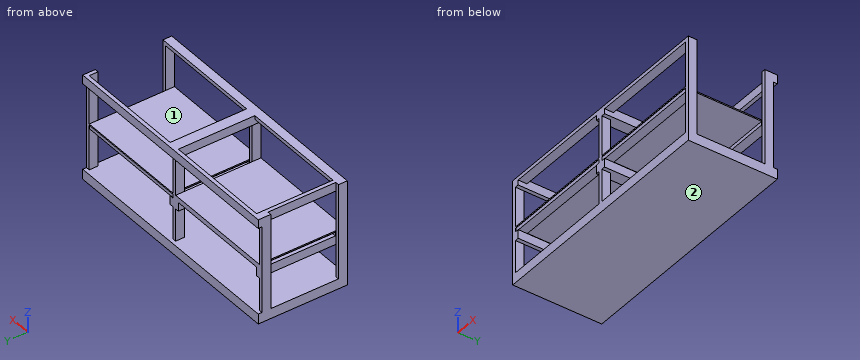
from build123d import *

# Parameters (mm, degrees)
F0_W           = 38.1
F0_H           = 88.9
F1_DEPTH       = 101.6
F2_DEPTH       = 927.1
F3_W           = 2438.4
F3_H           = 88.9
F4_DEPTH       = 38.1
F5_DEPTH       = 965.2
F6_W           = 2438.4
F6_H           = 88.9
F7_DEPTH       = 38.1
F8_W           = 88.9
F8_H           = 50.8
F9_DEPTH       = 38.1
F8_H_2         = 38.1
F8_W_2         = 3.175
F8_W_3         = 85.725
F10_DEPTH      = 1162.05
F11_W          = 863.6
F11_H          = 88.9
F12_DEPTH      = 38.1
F12_DEPTH_BACK = 76.2
F13_W          = 88.9
F13_H          = 38.1
F14_DEPTH      = 1162.05


with BuildPart() as f1:
    # F0 (on Top) → F1 (new body)
    with BuildSketch(Plane.XY):
        Polygon((38.1, 88.9), (38.1, 0), (1200.15, 0), (1200.15, 88.9), (1238.25, 88.9), (1238.25, 0), (2400.3, 0), (2400.3, 88.9), (2438.4, 88.9), (2438.4, 774.7), (2400.3, 774.7), (2400.3, 863.6), (1238.25, 863.6), (1238.25, 774.7), (1200.15, 774.7), (1200.15, 863.6), (38.1, 863.6), (38.1, 774.7), (0, 774.7), (0, 88.9), align=None)
        with Locations((19.05, 819.15)):
            Rectangle(F0_W, F0_H)
        with Locations((1219.2, 819.15)):
            Rectangle(F0_W, F0_H)
        with Locations((2419.35, 819.15)):
            Rectangle(F0_W, F0_H)
        with Locations((2419.35, 44.45)):
            Rectangle(F0_W, F0_H)
        with Locations((1219.2, 44.45)):
            Rectangle(F0_W, F0_H)
        with Locations((19.05, 44.45)):
            Rectangle(F0_W, F0_H)
        Polygon((0, 901.7), (0, 863.6), (38.1, 863.6), (1200.15, 863.6), (1238.25, 863.6), (2400.3, 863.6), (2438.4, 863.6), (2438.4, 901.7), align=None)
    extrude(amount=-F1_DEPTH)

    # F0 (on Top) → F2 (join)
    with BuildSketch(Plane.XY):
        with Locations((19.05, 44.45)):
            Rectangle(F0_W, F0_H)
        with Locations((2419.35, 44.45)):
            Rectangle(F0_W, F0_H)
        with Locations((1219.2, 44.45)):
            Rectangle(F0_W, F0_H)
    extrude(amount=F2_DEPTH)

    # F3 (on face) → F4 (join)
    with BuildSketch(Plane.XY.offset(927.1)):
        with Locations((1219.2, 44.45)):
            Rectangle(F3_W, F3_H)
    extrude(amount=F4_DEPTH)

    # F0 (on Top) → F5 (join)
    with BuildSketch(Plane.XY):
        with Locations((19.05, 819.15)):
            Rectangle(F0_W, F0_H)
        with Locations((1219.2, 819.15)):
            Rectangle(F0_W, F0_H)
        with Locations((2419.35, 819.15)):
            Rectangle(F0_W, F0_H)
    extrude(amount=F5_DEPTH)

    # F6 (on face) → F7 (join)
    with BuildSketch(Plane(origin=(0, 863.6, 0), x_dir=(-1, 0, 0), z_dir=(0, 1, 0))):
        with Locations((-1219.2, 920.75)):
            Rectangle(F6_W, F6_H)
    extrude(amount=F7_DEPTH)

    # F8 (on face) → F9 (join)
    with BuildSketch(Plane.YZ.offset(38.1)):
        with Locations((44.45, 901.7)):
            Rectangle(F8_W, F8_H)
        Polygon((863.6, 965.2), (0, 965.2), (0, 927.1), (88.9, 927.1), (88.9, 876.3), (863.6, 876.3), align=None)
        Polygon((3.175, 419.1), (0, 419.1), (0, 330.2), (88.9, 330.2), (88.9, 419.1), align=None)
        Polygon((92.075, 419.1), (88.9, 419.1), (88.9, 330.2), (863.6, 330.2), (863.6, 419.1), (774.7, 419.1), align=None)
    extrude(amount=F9_DEPTH)

    # F8 (on face) → F10 (join, through all)
    with BuildSketch(Plane.YZ.offset(38.1)):
        Polygon((88.9, 469.9), (0, 469.9), (0, 457.2), (3.175, 457.2), (88.9, 457.2), align=None)
        Polygon((863.6, 469.9), (88.9, 469.9), (88.9, 457.2), (92.075, 457.2), (774.7, 457.2), (863.6, 457.2), align=None)
        with Locations((819.15, 438.15)):
            Rectangle(F8_W, F8_H_2)
        with Locations((90.4875, 438.15)):
            Rectangle(F8_W_2, F8_H_2)
        with Locations((46.0375, 438.15)):
            Rectangle(F8_W_3, F8_H_2)
    extrude(amount=F10_DEPTH)

    # F11 (on face) → F12 (join, two sides)
    with BuildSketch(Plane.YZ.offset(1238.25)) as f12_sk:
        with Locations((431.8, 920.75)):
            Rectangle(F11_W, F11_H)
        with Locations((431.8, 374.65)):
            Rectangle(F11_W, F11_H)
    extrude(amount=F12_DEPTH)
    extrude(f12_sk.sketch, amount=-F12_DEPTH_BACK)

    # F13 (on face) → F14 (join, through all)
    with BuildSketch(Plane.YZ.offset(1238.25)):
        Polygon((863.6, 469.9), (0, 469.9), (0, 457.2), (3.175, 457.2), (92.075, 457.2), (771.525, 457.2), (860.425, 457.2), (863.6, 457.2), align=None)
        with Locations((47.625, 438.15)):
            Rectangle(F13_W, F13_H)
        with Locations((815.975, 438.15)):
            Rectangle(F13_W, F13_H)
    extrude(amount=F14_DEPTH)


solid = f1.part
CAD build for the part. Positions are in the model's coordinates, mm. Face numbers are marked on the shaded views. Round coordinates to 2 decimals unless told otherwise and drop trailing zeros. Order: outer loops, then holes, each group sorted by start corner. A loop starts at its lowest first (then second) coordinate and runs counter-clockwise, first axis right, second up. Notation, with made-up numbers: (12.25, -30.5) -> (58.25, -30.5) arc R31 cw to (58.25, -5.5) -> close; hole circle Ø6 at (83, 80.5). An arc over 180 degrees is marked (long way). Write item = value, one per line. Start each with the question number.
(1) Pin check, flat tips, straight feed: P1, Ø5, axis at y = 247, z = 406.5, coming from the -X side; P2, Ø5, axis at x = 310.5, y = 369, coming from the +Z side; P3, Ø19, axis at x = 1672.5, z = 432, coming from the -Y side (3 decimals). Stop position of each tip, or through.
(2) Cut at A-A, the plane y = 520. List the corners of the cut face in (x, z), then the cut area to 3 significant figures.
(3) Pull direction X, two halves, no side cores. Call the marked faces 1 and 2: released by +X, released by -X, zero draft, split by the parting line, or undercut.
(4) Cut at B-B, the plane x = 1717. List the corners of the cut face in (y, z) (3 decimals), then the cut area to 3 significant figures.
(5) Probe line 1 (X direction, y = 36, z = 19.5); line 2 (Z direction, x = 483.5, y = 335); line 3 (Z direction, x = 1664, y = 832.5). List the from-to ranges inside material, lowest first. Write a range as [from, to].
(6) Cut at D-D, the plane y = 818. State how many separate pieces and enclosed holes the cut face has, then the cut area to 3 significant figures.
(7) Cut at C-C, the plane z = 354. List the corners of the cut face in (x, y).
Model answer:
q1.P1 = 38.1
q1.P2 = 469.9
q1.P3 = 3.175
q2.outline = (0, -101.6) -> (2438.4, -101.6) -> (2438.4, 0) -> (0, 0) -> close; (38.1, 330.2) -> (76.2, 330.2) -> (76.2, 419.1) -> (38.1, 419.1) -> close; (38.1, 457.2) -> (1200.15, 457.2) -> (1200.15, 469.9) -> (38.1, 469.9) -> close; (38.1, 876.3) -> (76.2, 876.3) -> (76.2, 965.2) -> (38.1, 965.2) -> close; (1162.05, 330.2) -> (1276.35, 330.2) -> (1276.35, 419.1) -> (1162.05, 419.1) -> close; (1162.05, 876.3) -> (1276.35, 876.3) -> (1276.35, 965.2) -> (1162.05, 965.2) -> close; (1238.25, 457.2) -> (2400.3, 457.2) -> (2400.3, 469.9) -> (1238.25, 469.9) -> close
q2.area = 304,000 mm2
q3.face_1 = undercut
q3.face_2 = zero draft
q4.outline = (0, -101.6) -> (901.7, -101.6) -> (901.7, 0) -> (0, 0) -> close; (0, 457.2) -> (3.175, 457.2) -> (3.175, 419.1) -> (92.075, 419.1) -> (92.075, 457.2) -> (771.525, 457.2) -> (771.525, 419.1) -> (860.425, 419.1) -> (860.425, 457.2) -> (863.6, 457.2) -> (863.6, 469.9) -> (0, 469.9) -> close; (0, 927.1) -> (88.9, 927.1) -> (88.9, 965.2) -> (0, 965.2) -> close; (863.6, 876.3) -> (901.7, 876.3) -> (901.7, 965.2) -> (863.6, 965.2) -> close
q4.area = 116,000 mm2
q5.line_1 = [0, 38.1], [1200.15, 1238.25], [2400.3, 2438.4]
q5.line_2 = [-101.6, 0], [457.2, 469.9]
q5.line_3 = [-101.6, 0], [419.1, 469.9]
q6.separate_pieces = 1
q6.enclosed_holes = 2
q6.area = 496,000 mm2
q7.outline = (0, 0) -> (76.2, 0) -> (76.2, 863.6) -> (0, 863.6) -> (0, 774.7) -> (38.1, 774.7) -> (38.1, 88.9) -> (0, 88.9) -> close; (1162.05, 0) -> (1276.35, 0) -> (1276.35, 863.6) -> (1162.05, 863.6) -> close; (2400.3, 0) -> (2438.4, 0) -> (2438.4, 88.9) -> (2400.3, 88.9) -> close; (2400.3, 774.7) -> (2438.4, 774.7) -> (2438.4, 863.6) -> (2400.3, 863.6) -> close
